CAD build for the part. Positions are in the model's coordinates, mm. Face numbers are marked on the shaded views. Give positions to 0.01 mm unless a question says otherwise; leave off trailing zeros. Loops run counter-clockwise (first coordinate to the right, second up) from the corner with the lowest first, then second, coordinate; pieces in that order, holes last. Notation, with made-up numbers: (65, 22) -> (83, 22) arc R18 cw to (83, 36) -> close; hole circle Ø1 at (20.25, 50). An arc over 180 degrees is marked (long way). Use one line per item in the form item = value.
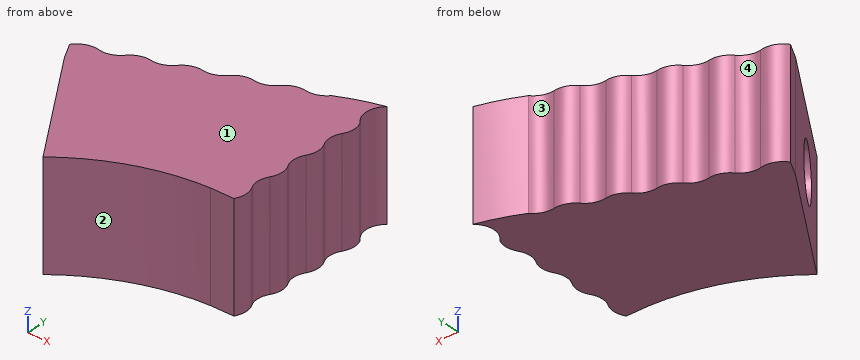
Autodesk Inventor part; units mm, degrees
ref_plane "YZ Plane" through (0, 0, 0) normal (1, 0, 0) x (0, 1, 0)
ref_plane "XZ Plane" through (0, 0, 0) normal (0, 1, 0) x (-1, 0, 0)
ref_plane "XY Plane" through (0, 0, 0) normal (0, 0, 1) x (1, 0, 0)
sketch "Sketch1" plane through (0, 0, 0) normal (0, 0, 1) x (1, 0, 0)
  line L0 (0, 0) -> (-1.6764, 0)
  line L1 (-2.8195, 0) -> (-2.8195, -0.0085)
  arc A0 (-2.8195, -0.0085) -> (-18.0949, -6.0198) centre (-1.6549, -25.3818) ccw
  line L2 (-28.1765, 8.5246) -> (-18.0949, -6.0198)
  line L3 (-28.1765, 8.5246) -> (-29.3649, 10.6117)
  line L4 (-17.1011, 15.221) -> (-17.0941, 15.2016)
  line L5 (-9.9296, 17.7969) -> (-9.9234, 17.7799)
  line L6 (-7.5786, 18.7636) -> (-7.5777, 18.7612)
  line L7 (-2.8195, -0.0085) -> (0, 0)
  line L8 (-0.0077, 2.54) -> (0, 0)
  arc A1 (-26.6104, 11.642) -> (-29.3649, 10.6117) centre (-27.262, 9.187) ccw
  arc A2 (-26.6104, 11.642) -> (-24.2313, 12.5319) centre (-26.1915, 14.1472) ccw
  arc A3 (-21.8523, 13.4218) -> (-24.2313, 12.5319) centre (-22.2712, 10.9166) ccw
  arc A4 (-21.8523, 13.4218) -> (-19.4732, 14.3117) centre (-21.4333, 15.927) ccw
  arc A5 (-17.1011, 15.221) -> (-19.4732, 14.3117) centre (-17.4998, 12.7125) ccw
  arc A6 (-17.1011, 15.221) -> (-14.715, 16.0915) centre (-16.6619, 17.7227) ccw
  arc A7 (-12.3359, 16.9814) -> (-14.715, 16.0915) centre (-12.7548, 14.4762) ccw
  arc A8 (-12.3359, 16.9814) -> (-9.9568, 17.8713) centre (-11.917, 19.4866) ccw
  arc A9 (-7.5786, 18.7636) -> (-9.9568, 17.8713) centre (-7.9949, 16.258) ccw
  arc A10 (-7.5786, 18.7636) -> (-5.1986, 19.6511) centre (-7.1571, 21.2684) ccw
  arc A11 (-0.065, 21.5463) -> (-5.1986, 19.6511) centre (6.1141, -3.0906) ccw
  arc A12 (-0.065, 21.5463) -> (-0.0536, 17.7799) centre (1.6451, 19.6683) ccw
  arc A13 (-0.046, 15.2399) -> (-0.0536, 17.7799) centre (-2.2495, 16.5033) ccw
  arc A14 (-0.046, 15.2399) -> (-0.0383, 12.6999) centre (2.1575, 13.9766) ccw
  arc A15 (-0.0307, 10.16) -> (-0.0383, 12.6999) centre (-2.2342, 11.4233) ccw
  arc A16 (-0.0307, 10.16) -> (-0.023, 7.62) centre (2.1729, 8.8966) ccw
  arc A17 (-0.0153, 5.08) -> (-0.023, 7.62) centre (-2.2189, 6.3433) ccw
  arc A18 (-0.0153, 5.08) -> (-0.0077, 2.54) centre (2.1882, 3.8166) ccw
  arc A19 (0, 0) -> (-0.0077, 2.54) centre (-2.2035, 1.2634) ccw
  line L9 (-0.275, 21.4927) -> (-0.0651, 21.5712)
  line L10 (-7.5777, 18.7612) -> (-7.5734, 18.7628)
  line L11 (-29.3649, 10.6117) -> (-26.6104, 11.642)
  line L12 (-17.0941, 15.2016) -> (-17.0604, 15.2142)
  line L13 (-0.0651, 21.5712) -> (-0.065, 21.5463)
  line L14 (-0.0077, 2.54) -> (0, 0)
  line L15 (-2.8195, 0) -> (-2.8195, 3.7275)
  dimension "d14" = 10.6117
  dimension "d15" = 29.3649
  dimension "d21" = 21.5712
  dimension "d22" = 29.2998
  dimension "d25" = 6.0198
  dimension "d26" = 18.0949
  dimension "d27" = 0
  dimension "d30" = 2.54
  dimension "d40" = 2.54
  dimension "d41" = 2.54
  dimension "d42" = 2.54
  dimension "d43" = 2.54
  dimension "d44" = 2.54
  dimension "d45" = 2.54
  dimension "d46" = 2.54
  dimension "d47" = 2.54
  dimension "d48" = 2.54
  dimension "d49" = 2.54
  dimension "d50" = 25.4
  dimension "d51" = 2.54
  dimension "d52" = 2.54
  dimension "d53" = 2.54
  dimension "d54" = 2.54
  dimension "d55" = 2.54
  dimension "d56" = 2.54
  dimension "d57" = 2.54
  dimension "d58" = 2.54
extrude "Extrusion1" add sketch "Sketch1" along normal blind 12.7 contours A0 L2 L3 L11 A2 A3 A4 A5 L4 L12 A6 A7 A8 A9 L6 L10 A10 A11 A12 A13 A14 A15 A16 A17 A18 L8 L7 | L8 A19 | A1 L11
sketch "Sketch2" plane through (-18.0949, -6.0198, 0) normal (-0.8219, -0.5697, 0) x (0, 0, 1)
  line L0 (0, 17.6968) -> (0, 0)
  line L1 (12.7, 17.751) -> (0, 17.751)
  line L2 (0, 17.751) -> (0, 0)
  line L3 (0, 0) -> (12.7, 0)
  line L4 (12.7, 0) -> (12.7, 17.751)
  line L5 (12.7, 0.1215) -> (0, 0.1215)
  line L6 (12.7, 17.751) -> (6.35, 17.751)
  line L7 (6.35, 17.751) -> (6.35, 0.1215)
  line L8 (6.35, 0.1215) -> (12.7, 0.1215)
  line L9 (12.7, 0.1215) -> (12.7, 17.751)
  circle A0 centre (6.35, 7.7415) radius 3.175
  point P0 (0, -5.3609)
  dimension "d62" = 6.35
  dimension "d63" = 7.62
extrude "Extrusion2" cut sketch "Sketch2" against normal blind 19.05 contours A0 L7 | L7 A0
properties part number "tippa dis claw"
1. Mould opens along X. For the marked faces 1, 2, 3 and 4 say: pulls with the +X half, pulls with the -X half, needs draft (parallel to the pull), parting line crosses it, or undercut.
Result sheet:
face_1 = needs draft
face_2 = pulls with the +X half
face_3 = undercut
face_4 = undercut
2. Cut at B-B, the plane y = -3.25. Write the cut outline in (x, z), then the cut area to 3 significant figures.
Result sheet:
outline = (-20.01, 0) -> (-14.12, 0) -> (-14.12, 12.7) -> (-20.01, 12.7) -> close
area = 74.9 mm^2
3. Drill centre lines: line 1 (X direction, y = 10, z = 5); line 2 (X direction, y = 4.25, z = 8.25); line 3 (Y direction, x = -5.75, z = 6.25). Where is each one in solid material? Low to high.
Result sheet:
line_1 = -29.02 to -13.62, -6.02 to -0.12
line_2 = -25.21 to -21.33, -12.4 to -0.31
line_3 = -0.31 to 8.1, 9.61 to 19.15
4. Cut at C-C, the plane x = -1.25. Write the cut outline in (y, z).
Result sheet:
outline = (0, 0) -> (21.22, 0) -> (21.22, 12.7) -> (0, 12.7) -> close
5. Drop a flat-ended pin along its axis: P1, Ø2, axis at y = 15, z = 1.5, coming from the -X side. Give the stop position or say it passes through.
Result sheet:
P1 = -19.78
